Check sheet for the modelled part. Datum: model origin and axes. Units: mm. A direction names the side the tool comes from. Coordinates: 2 decimals unless noted, no trailing zeros. Write each loop counter-clockwise with the first axis right and the second up, starting at its lowest first coordinate (ties: lowest second). Pieces come first, ordered by that corner, then holes. Notation, with made-up numbers: (34, 33) -> (67, 33) arc R3 ccw to (67, 37) -> close; hole circle Ø1 at (-23.5, 73). An arc over 180 degrees is marked (long way). Put each result on its own line as item: value.
```python
from build123d import *

# Parameters (mm, degrees)
SKETCH1_R           = 14
BOSS_EXTRUDE1_DEPTH = 15.5
CHAMFER1_SIZE       = 2.54
CHAMFER1_SIZE2      = 4.399409051
SKETCH2_R           = 1.5875
BOSS_EXTRUDE2_DEPTH = 14.1


with BuildPart() as part:
    # Sketch1 → Boss-Extrude1 (new body, symmetric)
    with BuildSketch(Plane(origin=(0, 0, 0), x_dir=(1, 0, 0), z_dir=(0, 1, 0))):
        Circle(SKETCH1_R)
    extrude(amount=BOSS_EXTRUDE1_DEPTH, both=True)

    # Chamfer1
    chamfer1_edges = [part.edges().sort_by_distance(p)[0] for p in [
        (-14, 15.5, 0),
    ]]
    chamfer1_side = [part.faces().sort_by_distance(p)[0] for p in [
        (-14, 0, 0),
    ]]
    chamfer(chamfer1_edges, length=CHAMFER1_SIZE, length2=CHAMFER1_SIZE2, reference=chamfer1_side[0])

    # Sketch2 → Boss-Extrude2 (add)
    with BuildSketch(Plane.XZ.offset(15.5)):
        Circle(SKETCH2_R)
    extrude(amount=BOSS_EXTRUDE2_DEPTH)


solid = part.part
```
Q1. Depth check by flat-ended pin: P1, Ø2, axis at x = 3.5, y = 8, coming from the -Z side (3 decimals); P2, Ø2, axis at x = 8.5, y = 0, coming from the +Z side; P3, Ø5, axis at x = -7.5, z = -11, coming from the -Y side. Enter the tip coordinate at first touch or a pass-through.
Recorded:
P1: stops at z = -13.775
P2: stops at z = 11.82
P3: stops at y = -15.5
Q2. Material ranges on line 1 along Y through (x, z) = (-9, -0.25); line 2 along X through (y, z) = (-3, -3.5); line 3 along Z through (x, y) = (-6.5, -7.5), recorded low to high.
Recorded:
line 1: y = -15.5 to 15.5
line 2: x = -13.56 to 13.56
line 3: z = -12.4 to 12.4
Q3. Tool access check on faces 1 (the cylindrical face through (-0.34, -22.45, -1.55)), 2 (the flat face through (0, -29.6, 0)). Record the directions out of +Z, -Z, +X, -X, +Y, -Y that give a thin tool (end or side, any length) a straight path to the whole face; none if there is none.
Recorded:
face 1: -Y
face 2: +Z, -Z, +X, -X, -Y
Q4. Cross-section at C-C (y = 8). Record the cut outline in (x, z).
Recorded:
outline: circle Ø28 at (0, 0)
Q5. Cross-section at B-B (x = 0). Record the cut outline in (y, z), plus the area to 3 significant figures.
Recorded:
outline: (-29.6, -1.59) -> (-15.5, -1.59) -> (-15.5, -14) -> (12.96, -14) -> (15.5, -9.6) -> (15.5, 9.6) -> (12.96, 14) -> (-15.5, 14) -> (-15.5, 1.59) -> (-29.6, 1.59) -> close
area: 902 mm2
Q6. Cross-section at A-A (z = 0). Record the cut outline in (x, y).
Recorded:
outline: (-14, -15.5) -> (-1.59, -15.5) -> (-1.59, -29.6) -> (1.59, -29.6) -> (1.59, -15.5) -> (14, -15.5) -> (14, 12.96) -> (9.6, 15.5) -> (-9.6, 15.5) -> (-14, 12.96) -> close
